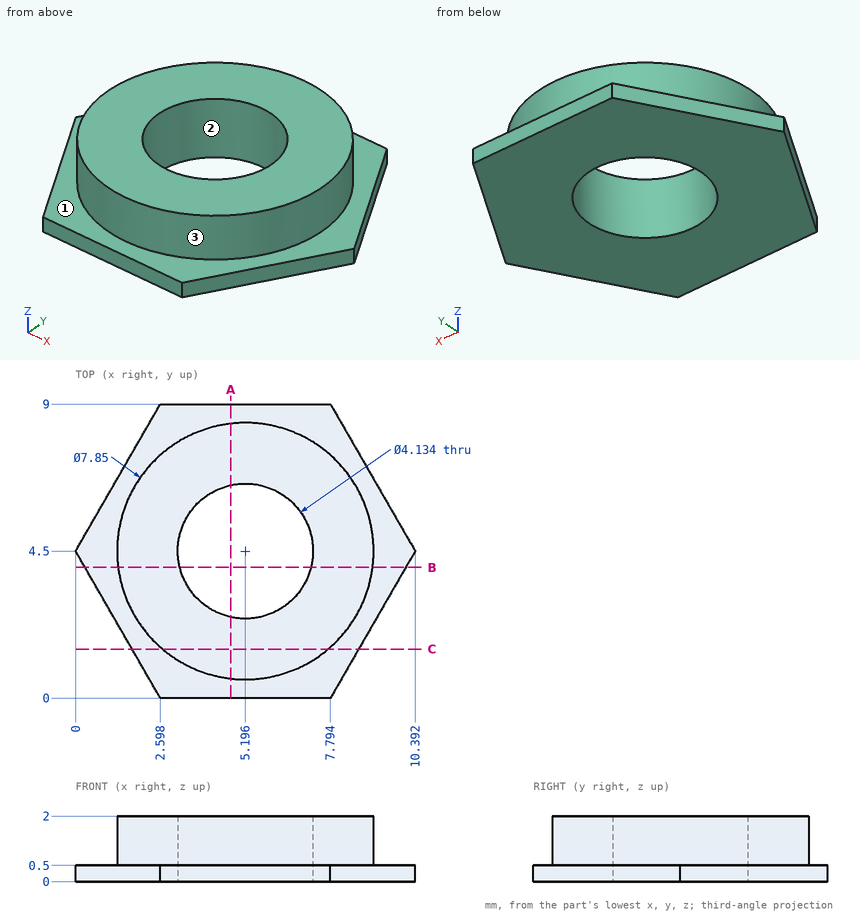
Study the drawing (mm; zero at the part's minimum x, y, z) and answer. Coordinates: 2 decimals unless noted, no trailing zeros. Loops run counter-clockwise (first coordinate to the right, second up) from the corner with the lowest first, then second, coordinate; pieces in that order, holes last. Notation, with made-up numbers: (60.25, 86.25) -> (111.25, 86.25) arc R11 cw to (111.25, 92.25) -> close; hole circle Ø6 at (61, 80). An arc over 180 degrees is marked (long way). Answer as CSV lines item,"result".
1) The part is cut by section C-C (y = 1.5). Give the vertices of the cut face in (x, z) (1 decimal).
A:
outline,"(1.7, 0) -> (8.7, 0) -> (8.7, 0.5) -> (7.7, 0.5) -> (7.7, 2) -> (2.7, 2) -> (2.7, 0.5) -> (1.7, 0.5) -> close"
2) A flat-ended cylindrical pin translates along its axis: pin 1 (2.5 mm diameter, centred on x = 6.5, y = 6, fed in from +Z). Find the tip coordinate at first contact, or state that the pin passes through.
A:
pin 1,"stops at z = 2"
3) The part is cut by section B-B (y = 4). Give the vertices of the cut face in (x, z).
A:
outline,"(0.29, 0) -> (3.19, 0) -> (3.19, 2) -> (1.3, 2) -> (1.3, 0.5) -> (0.29, 0.5) -> close; (7.2, 0) -> (10.1, 0) -> (10.1, 0.5) -> (9.09, 0.5) -> (9.09, 2) -> (7.2, 2) -> close"
4) Straight lines are drawn through the part: probe 1 along Y at (x, z) = (4.5, 1.6) (1 decimal); probe 2 along Z at (x, y) = (3.75, 0.5); probe 3 along X at (y, z) = (5.5, 0.85) (1 decimal). For each, find the intervals that lie inside material, in ascending order.
A:
probe 1,"y = 0.6 to 2.6, 6.4 to 8.4"
probe 2,"z = 0 to 0.5"
probe 3,"x = 1.4 to 3.4, 7 to 9"
5) For a pull along Y with two mould halves and no side action, classify the marked faces 1, 2 and 3 as released by +Y, released by -Y, zero draft, split by the parting line, or undercut.
A:
face 1,"zero draft"
face 2,"undercut"
face 3,"split by the parting line"
6) The part is cut by section A-A (x = 4.75). Give the vertices of the cut face in (y, z).
A:
outline,"(0, 0) -> (2.48, 0) -> (2.48, 2) -> (0.6, 2) -> (0.6, 0.5) -> (0, 0.5) -> close; (6.52, 0) -> (9, 0) -> (9, 0.5) -> (8.4, 0.5) -> (8.4, 2) -> (6.52, 2) -> close"
